For this review, use the dimensioned drawing (mm, ordinates from the lowest corner) and the shaded views. A direction names the side the tool comes from. Round coordinates to 2 decimals unless told otherwise and drop trailing zeros. Loops run counter-clockwise (first coordinate to the right, second up) from the corner with the lowest first, then second, coordinate; pieces in that order, holes last. Notation, with made-up numbers: (7, 70) - (29, 70) arc R22 cw to (29, 105) - close; hole circle Ø1 at (65.25, 59.5). An arc over 180 degrees is marked (long way). One line per question, with ' | ' between items. Start each with the question number.
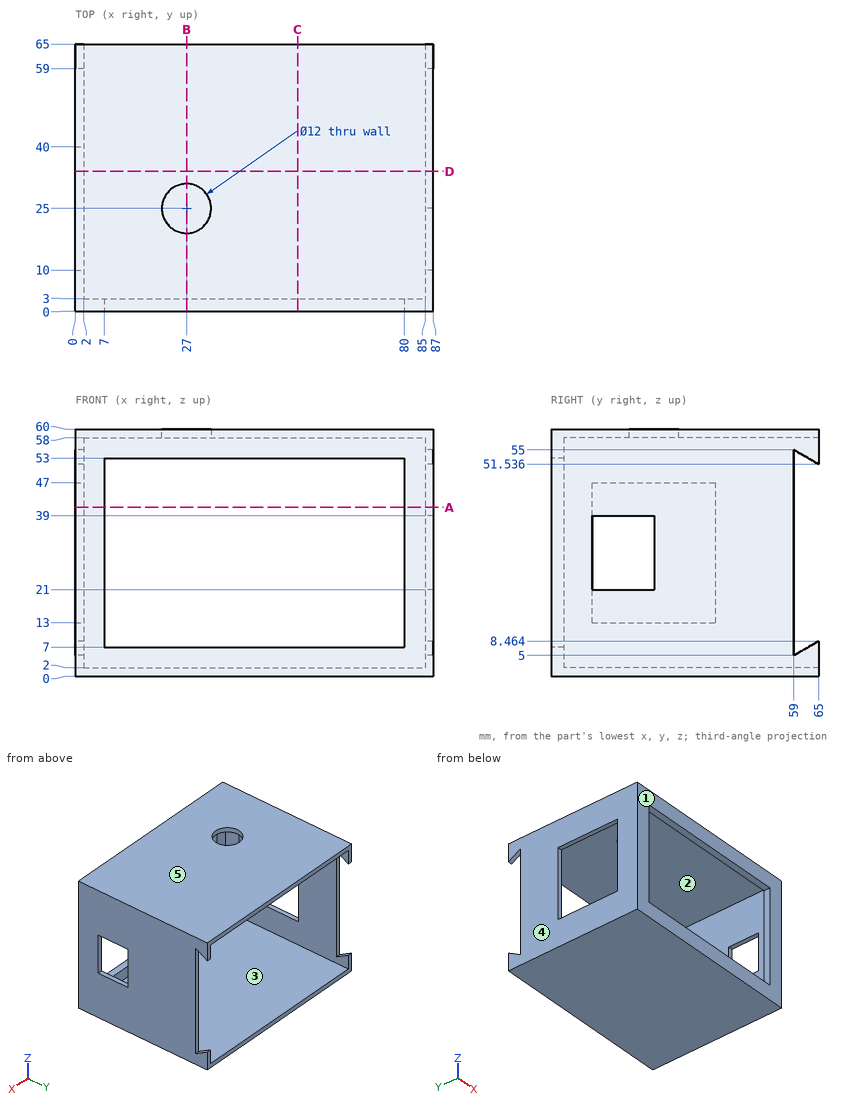
1. To check wall thickness, follow line 1 along Y through (x, z) = (27, 58.75); line 2 along Z through (x, y) = (62.5, 14.5); line 3 along X through (y, z) = (5, 55). State the ranges of each line that lie inside material, in increasing order.
2. Take a section at C-C, the plane x = 54. Give the boundary of the cut face in (y, z), then the cut area to 3 significant figures.
3. Clearance check with flat-ended pins moving along their axes: P1, Ø1.6, axis at x = 86, y = 17.5, coming from the -Z side; P2, Ø10, axis at y = 31, z = 40, coming from the -X side; P3, Ø2, axis at x = 1, z = 34, coming from the +Y side. State where each tip first meets the part, or that it passes through.
4. Take a section at B-B, the plane x = 27. Give the boundary of the cut face in (y, z), then the cut area to 3 significant figures.
5. Machinability: for the marked faces 1 and 2, which of the approach directions +Z, -Z, +X, -X, +Y, -Y give a long, thin tool a straight path to every point of the face, cutting with its end or side? Answer none if there is none.
6. Take a section at D-D, the plane y = 34. Give the boundary of the cut face in (x, z).
7. Take a section at A-A, the plane z = 41. Give the boundary of the cut face in (x, y).
8. The part is to be moulded in two halves that separate along Z. For the marked faces 3, 4 and 5, say which applies: pulls with the +Z half, pulls with the -Z half, needs draft (parallel to the pull), parting line crosses it, or undercut.
Answer list:
1) line 1: y = 0 to 19, 31 to 65 | line 2: z = 0 to 2, 58 to 60 | line 3: x = 0 to 2, 85 to 87
2) outline: (0, 0) - (65, 0) - (65, 2) - (3, 2) - (3, 7) - (0, 7) - close; (0, 53) - (3, 53) - (3, 58) - (65, 58) - (65, 60) - (0, 60) - close | area: 290 mm²
3) P1: stops at z = 0 | P2: stops at x = 85 | P3: stops at y = 59
4) outline: (0, 0) - (65, 0) - (65, 2) - (3, 2) - (3, 7) - (0, 7) - close; (0, 53) - (3, 53) - (3, 58) - (19, 58) - (19, 60) - (0, 60) - close; (31, 58) - (65, 58) - (65, 60) - (31, 60) - close | area: 266 mm²
5) face 1: +Z, -Z, +X, -X, -Y | face 2: +Y
6) outline: (0, 0) - (87, 0) - (87, 60) - (0, 60) - (0, 47) - (2, 47) - (2, 58) - (85, 58) - (85, 2) - (2, 2) - (2, 13) - (0, 13) - close
7) outline: (0, 0) - (7, 0) - (7, 3) - (2, 3) - (2, 10) - (0, 10) - close; (0, 40) - (2, 40) - (2, 59) - (0, 59) - close; (80, 0) - (87, 0) - (87, 59) - (85, 59) - (85, 3) - (80, 3) - close
8) face 3: undercut | face 4: needs draft | face 5: pulls with the +Z half
